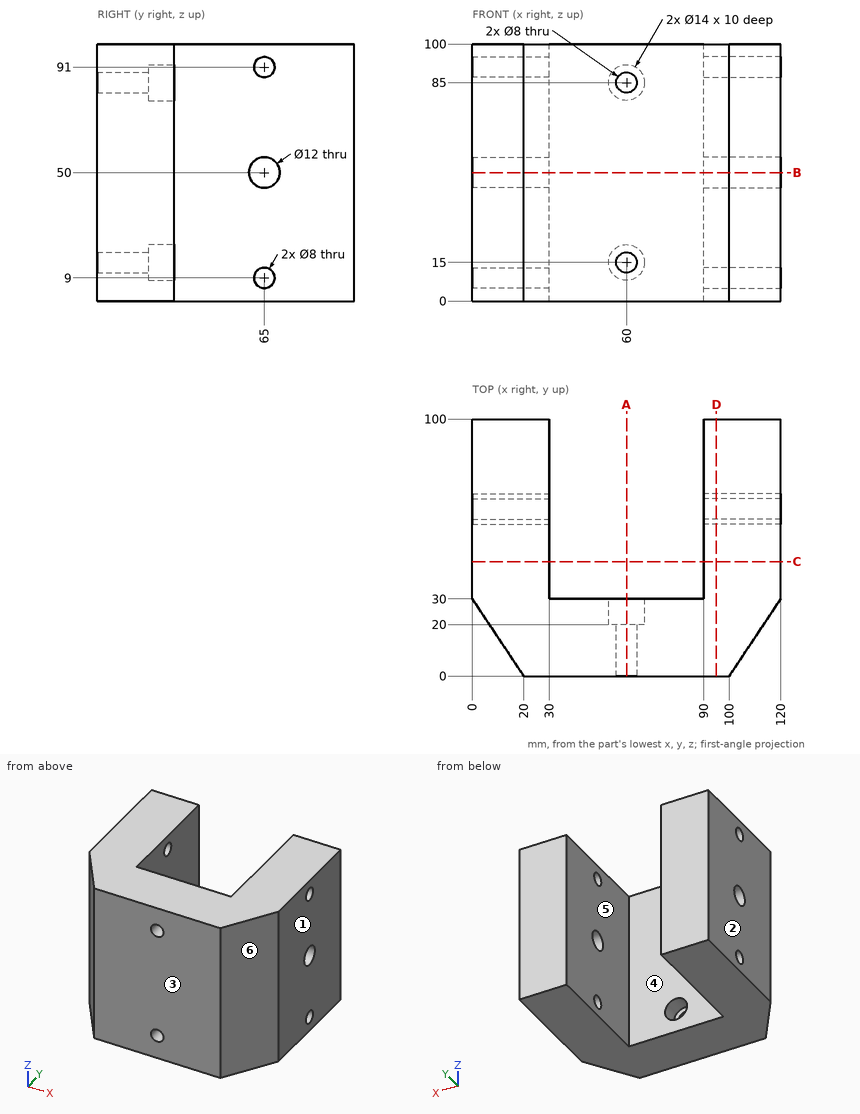
Geometry: see drawing. Coordinates: mm, zero at the bounding-box minimum. A direction names the side the tool comes from. Coordinates: 2 decimals unless noted, no trailing zeros. Loops run counter-clockwise (first coordinate to the right, second up) from the corner with the lowest first, then second, coordinate; pieces in that order, holes last. Notation, with made-up numbers: M 50.25,-10 L 59.25,-10 A10 ccw 59.25,3 Z; hole C 60.25,73 d11. An arc over 180 degrees is marked long. Answer in a Markdown table with one row per item.
Q1. Set-up query: the marked faces 5 and 6. Return all of +Z, -Z, +X, -X, +Y, -Y with unobstructed straight access to the full face (end or side cutting, diameter ignored); none if empty.
Answers below:
| item | result |
|---|---|
| face 5 | +Z, -Z, +Y |
| face 6 | +Z, -Z, +X, -Y |
Q2. Section A-A on x = 60. Return the cut outline in (y, z).
Answers below:
| item | result |
|---|---|
| outline | M 0,0 L 30,0 L 30,8 L 20,8 L 20,11 L 0,11 Z; M 0,19 L 20,19 L 20,22 L 30,22 L 30,78 L 20,78 L 20,81 L 0,81 Z; M 0,89 L 20,89 L 20,92 L 30,92 L 30,100 L 0,100 Z |
Q3. First-contact query: pin 1 (8 mm diameter, centred on y = 25.5, z = 57, fed in from +X); pin 2 (15.5 mm diameter, centred on x = 62, z = 83.5, fed in from +Y); pin 3 (12.5 mm diameter, centred on x = 60, z = 85, fed in from +Y). Flat tips, straight axial feed; report the tip coordinate or a pass-through.
Answers below:
| item | result |
|---|---|
| pin 1 | stops at x = 119.67 |
| pin 2 | stops at y = 30 |
| pin 3 | stops at y = 20 |
Q4. Section D-D on x = 95. Return the cut outline in (y, z).
Answers below:
| item | result |
|---|---|
| outline | M 0,0 L 100,0 L 100,100 L 0,100 Z; hole C 65,50 d12; hole C 65,9 d8; hole C 65,91 d8 |
Q5. Section C-C on y = 44.5. Return the cut outline in (x, z), plus the area to 3 significant figures.
Answers below:
| item | result |
|---|---|
| outline | M 0,0 L 30,0 L 30,100 L 0,100 Z; M 90,0 L 120,0 L 120,100 L 90,100 Z |
| area | 6,000 mm^2 |
Q6. Draft query along X for the marked faces 1, 2, 3 and 4. Return one class per face: pulls with the +X half, pulls with the -X half, needs draft (parallel to the pull), parting line crosses it, or undercut.
Answers below:
| item | result |
|---|---|
| face 1 | pulls with the +X half |
| face 2 | pulls with the -X half |
| face 3 | needs draft |
| face 4 | undercut |
Q7. Ray query, probe 1 along Z at (x, y) = (60, 24.25); probe 2 along Z at (x, y) = (97, 65); probe 3 along X at (y, z) = (76.5, 29). Return the intervals inside material, ascending. Write a range as from..to.
Answers below:
| item | result |
|---|---|
| probe 1 | z = 0..8, 22..78, 92..100 |
| probe 2 | z = 0..5, 13..44, 56..87, 95..100 |
| probe 3 | x = 0..30, 90..120 |
Q8. Section B-B on z = 50. Return the cut outline in (x, y).
Answers below:
| item | result |
|---|---|
| outline | M 0,30 L 20,0 L 100,0 L 120,30 L 120,59 L 90,59 L 90,30 L 30,30 L 30,59 L 0,59 Z; M 0,71 L 30,71 L 30,100 L 0,100 Z; M 90,71 L 120,71 L 120,100 L 90,100 Z |
